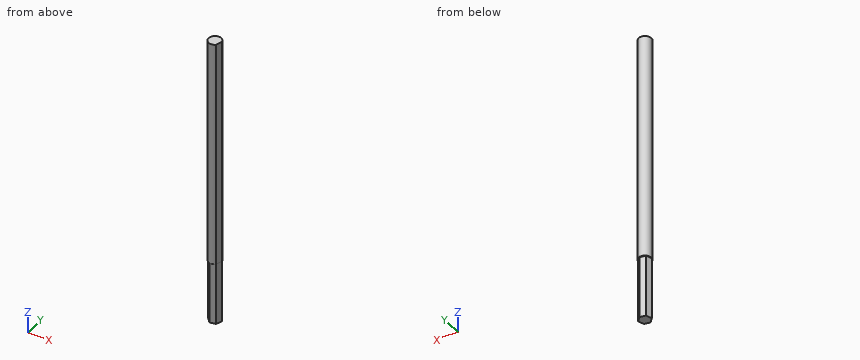
from build123d import *

# Parameters (mm, degrees)
SKETCH_1_R          = 3.05
EXTRUDE_1_DEPTH     = 110
EXTRUDE_2_DEPTH     = 30
SKETCH_3_W          = 148.461439859
SKETCH_3_H          = 21.991651446
CUT_EXTRUDE_1_DEPTH = 141.160128777


with BuildPart() as part:
    # 草图1 → 凸台-拉伸1 (new body)
    with BuildSketch(Plane.XY):
        Circle(SKETCH_1_R)
    extrude(amount=-EXTRUDE_1_DEPTH)

    # 草图2 → 凸台-拉伸2 (add)
    with BuildSketch(Plane(origin=(0, 0, -110), x_dir=(-1, 0, 0), z_dir=(0, 0, -1))):
        Polygon((1.953354878, 2.210634461), (-0.937788163, 2.796972178), (-2.891143041, 0.586337717), (-1.953354878, -2.210634461), (0.937788163, -2.796972178), (2.891143041, -0.586337717), align=None)
    extrude(amount=EXTRUDE_2_DEPTH)

    # 草图3 → 切除-拉伸1 (cut, through all)
    with BuildSketch(Plane(origin=(2.422248959, -0.812148372, 0), x_dir=(0, 0, -1), z_dir=(0.9481261618829849, -0.3178942924197286, 0))):
        with Locations((68.647762533, -0.511106719)):
            Rectangle(SKETCH_3_W, SKETCH_3_H)
    extrude(amount=CUT_EXTRUDE_1_DEPTH, mode=Mode.SUBTRACT)


solid = part.part
Build history of the part. All positions in model axes, mm. Give positions to 0.01 mm unless a question says otherwise; leave off trailing zeros. Order: outer loops, then holes, each group sorted by start corner. A loop starts at its lowest first (then second) coordinate and runs counter-clockwise, first axis right, second up. Notation, with made-up numbers: M 70,56.25 L 114,56.25 A30 ccw 114,89.25 Z; hole C 45,1 d6. An arc over 180 degrees is marked long. Use one line per item in the form item = value.
Q1. Wall check: probe 1 along Z at (x, y) = (-2.5, 1); probe 2 along X at (y, z) = (1.25, -84). Give the ranges that are in metal, low to high.
Conclusion:
probe_1 = -110 to 0
probe_2 = -2.78 to 2.78
Q2. Slice it at B-B, the plane z = -41.5. Write the cut outline in (x, y).
Conclusion:
outline = M 1.89,-2.39 L 2.95,0.77 A3.05 ccw long Z
Q3. Slice it at A-A, the plane x = 0. Write the cut outline in (y, z).
Conclusion:
outline = M -3.05,-110 L -2.61,-110 L -2.61,-140 L 2.61,-140 L 2.61,-110 L 3.05,-110 L 3.05,0 L -3.05,0 Z
